```python
from build123d import *

# Parameters (mm, degrees)
F1_DEPTH = 381
F2_R     = 55.1942
F3_R     = 55.1942
F4_T     = -6.35


with BuildPart() as f1:
    # F0 (on Top) → F1 (new body)
    with BuildSketch(Plane.XY):
        with BuildLine():
            Line((0, -215.9), (0, 215.9))
            ThreePointArc((0, 215.9), (-215.9, 0), (0, -215.9))
        make_face()
    extrude(amount=F1_DEPTH)

    # F2
    f2_edges = [f1.edges().sort_by_distance(p)[0] for p in [
        (-215.9, 0, 381),
    ]]
    fillet(f2_edges, radius=F2_R)

    # F3
    f3_edges = [f1.edges().sort_by_distance(p)[0] for p in [
        (-215.9, 0, 0),
    ]]
    fillet(f3_edges, radius=F3_R)

    # F4
    f4_openings = [f1.faces().sort_by_distance(p)[0] for p in [
        (0, 0, 190.5),
    ]]
    offset(amount=F4_T, openings=f4_openings)


solid = f1.part
```
Model file for the job. Use its own axes, mm. A direction names the side the tool comes from. Round coordinates to 2 decimals unless told otherwise and drop trailing zeros. Order: outer loops, then holes, each group sorted by start corner. A loop starts at its lowest first (then second) coordinate and runs counter-clockwise, first axis right, second up. Notation, with made-up numbers: (27, 88.5) -> (33, 88.5) arc R21 ccw to (33, 107.5) -> close; hole circle Ø2 at (31, 39). An arc over 180 degrees is marked (long way). Use one line per item in the form item = value.
Item 1: Cut at A-A, the plane z = 292. Write the cut outline in (x, y), and give its area (3 significant figures).
Returned:
outline = (0, -215.9) -> (0, -209.55) arc R209.55 cw to (0, 209.55) -> (0, 215.9) arc R215.9 ccw to start
area = 4,240 mm^2
Item 2: Pull direction Z, two halves, no side cores. Call faces 1 (the face through (-64, 2, 381)), 2 (the face through (-64, 2, 374.65)), 3 (the face through (-64, 2, 0)), 4 (the face through (-64, 2, 6.35)): released by +Z, released by -Z, zero draft, split by the parting line, or undercut.
Returned:
face_1 = released by +Z
face_2 = undercut
face_3 = released by -Z
face_4 = undercut
Item 3: Flat gauge pins, fed straight in: pin 1 Ø1.5 at (y, z) = (-92.5, 51.5) entering from +X; pin 2 Ø4 at (x, z) = (-163, 304.5) entering from -Y; pin 3 Ø2 at (x, y) = (-104, 145) entering from +Z; pin 4 Ø1 at (x, y) = (-74.5, -96) entering from -Z. Where does each tip first touch, or does it go through?
Returned:
pin_1 = -187.5
pin_2 = -143.85
pin_3 = 378.4
pin_4 = 0
Item 4: Drill centre lines: line 1 (Z direction, x = -119, y = -95); line 2 (Y direction, x = -151.5, z = 168.5); line 3 (Y direction, x = -127, z = 227.5). Where is each one in solid material? Low to high.
Returned:
line_1 = 0 to 6.35, 374.65 to 381
line_2 = -153.82 to -144.77, 144.77 to 153.82
line_3 = -174.6 to -166.68, 166.68 to 174.6
Item 5: Tool access for faces 5 (the face through (-215.848, 4.748, 188.606)), 6 (the face through (-209.5, 4.6, 188.6)): list every direction of +Z, -Z, +X, -X, +Y, -Y with a clear straight run to the whole face (end or side of a thin tool).
Returned:
face_5 = +Z, -Z, -X
face_6 = +X
Item 6: Cut at B-B, the plane z = 24.5. Write the cut outline in (x, y).
Returned:
outline = (0, -206.58) -> (0, -198.7) arc R198.7 cw to (0, 198.7) -> (0, 206.58) arc R206.58 ccw to start
